from build123d import *

# Parameters (mm, degrees)
F0_W     = 30
F0_H     = 30
F0_W_2   = 26
F0_H_2   = 26
F1_DEPTH = 2
F2_W     = 30
F2_H     = 30
F2_W_2   = 26.5
F2_H_2   = 26.2
F3_DEPTH = 4
F4_R     = 0.5
F5_W     = 15
F5_H     = 15
F6_DEPTH = 25


with BuildPart() as f1:
    # F0 (on Top) → F1 (new body)
    with BuildSketch(Plane.XY):
        Rectangle(F0_W, F0_H)
        Rectangle(F0_W_2, F0_H_2, mode=Mode.SUBTRACT)
        Rectangle(F0_W_2, F0_H_2)
    extrude(amount=F1_DEPTH)

    # F2 (on face) → F3 (join)
    with BuildSketch(Plane.XY.offset(2)):
        Rectangle(F2_W, F2_H)
        Rectangle(F2_W_2, F2_H_2, mode=Mode.SUBTRACT)
    extrude(amount=F3_DEPTH)

    # F4
    f4_edges = [f1.edges().sort_by_distance(p)[0] for p in [
        (-13.25, 0, 6),
        (0, 13.1, 6),
        (13.25, 0, 6),
        (0, -13.1, 6),
        (-13.25, 13.1, 4),
        (-13.25, -13.1, 4),
        (13.25, 13.1, 4),
        (13.25, -13.1, 4),
    ]]
    fillet(f4_edges, radius=F4_R)

    # F5 (on face) → F6 (cut)
    with BuildSketch(Plane.XY.offset(2)):
        Rectangle(F5_W, F5_H)
    extrude(amount=-F6_DEPTH, mode=Mode.SUBTRACT)


solid = f1.part
Could you check a few things on this model? Use its own coordinates, in mm. A direction names the side the tool comes from. Coordinates: 2 decimals unless noted, no trailing zeros. Order: outer loops, then holes, each group sorted by start corner. A loop starts at its lowest first (then second) coordinate and runs counter-clockwise, first axis right, second up.
Q1. Suppose I cut it at B-B on z = 2.6. Please give me the cut outline in (x, y).
Q2. Thinking about a two-plate mould opening in Y: for faces 1 (the flat face through (7.5, 0, 1)), 2 (the flat face through (0, -13.1, 4)), 3 (the flat face through (0, -15, 3)), 4 (the flat face through (-0.1, 14.5, 6)), which applies, released by +Y, released by -Y, zero draft, split by the parting line, or undercut?
Q3. Please list where these lines run through material, in increasing order: L1, parallel to Y at x = -5.25, z = 4.3; L2, parallel to Y at x = -2, z = 0.75; L3, parallel to X at y = -12.5, z = 3.5.
Q4. Suppose I cut it at D-D on x = 10.75. Please give me the cut outline in (y, z).
Q5. Which directions (+Z, -Z, +X, -X, +Y, -Y) give clear straight access to the entire face, cutting with the end or side of a thin tool? Please do faces 5 (the flat face through (-7.5, 0, 1)), 6 (the flat face through (0, 10, 0)), 7 (the flat face through (0, -9, 2)).
Q6. Suppose I cut it at C-C on x = 0.25. Please give me the cut outline in (y, z), and give its area (3 significant figures).
Q7. Will these pins go through, and if not, where does the flat tip stop? pin 1 (8 mm diameter, centred on x = -2.5, y = 5, fed in from +Z); pin 2 (4 mm diameter, centred on x = 1, y = -7.5, fed in from -Z).
Q8. Suppose I cut it at A-A on y = 0.5. Please give me the cut outline in (x, z), and give its area (3 significant figures).
Answer:
1. outline: (-15, -15) - (15, -15) - (15, 15) - (-15, 15) - close; hole (-13.25, -12.6) arc R0.5 ccw to (-12.75, -13.1) - (12.75, -13.1) arc R0.5 ccw to (13.25, -12.6) - (13.25, 12.6) arc R0.5 ccw to (12.75, 13.1) - (-12.75, 13.1) arc R0.5 ccw to (-13.25, 12.6) - close
2. face 1: undercut
2. face 2: undercut
2. face 3: released by -Y
2. face 4: zero draft
3. L1: y = -15 to -13.1, 13.1 to 15
3. L2: y = -15 to -7.5, 7.5 to 15
3. L3: x = -15 to -13.25, 13.25 to 15
4. outline: (-15, 0) - (15, 0) - (15, 6) - (13.6, 6) arc R0.5 ccw to (13.1, 5.5) - (13.1, 2) - (-13.1, 2) - (-13.1, 5.5) arc R0.5 ccw to (-13.6, 6) - (-15, 6) - close
5. face 5: +Z, -Z
5. face 6: -Z, +X, -X, +Y, -Y
5. face 7: +Z
6. outline: (-15, 0) - (-7.5, 0) - (-7.5, 2) - (-13.1, 2) - (-13.1, 5.5) arc R0.5 ccw to (-13.6, 6) - (-15, 6) - close; (7.5, 0) - (15, 0) - (15, 6) - (13.6, 6) arc R0.5 ccw to (13.1, 5.5) - (13.1, 2) - (7.5, 2) - close
6. area: 45.1 mm2
7. pin 1: stops at z = 2
7. pin 2: stops at z = 0
8. outline: (-15, 0) - (-7.5, 0) - (-7.5, 2) - (-13.25, 2) - (-13.25, 5.5) arc R0.5 ccw to (-13.75, 6) - (-15, 6) - close; (7.5, 0) - (15, 0) - (15, 6) - (13.75, 6) arc R0.5 ccw to (13.25, 5.5) - (13.25, 2) - (7.5, 2) - close
8. area: 43.9 mm2
